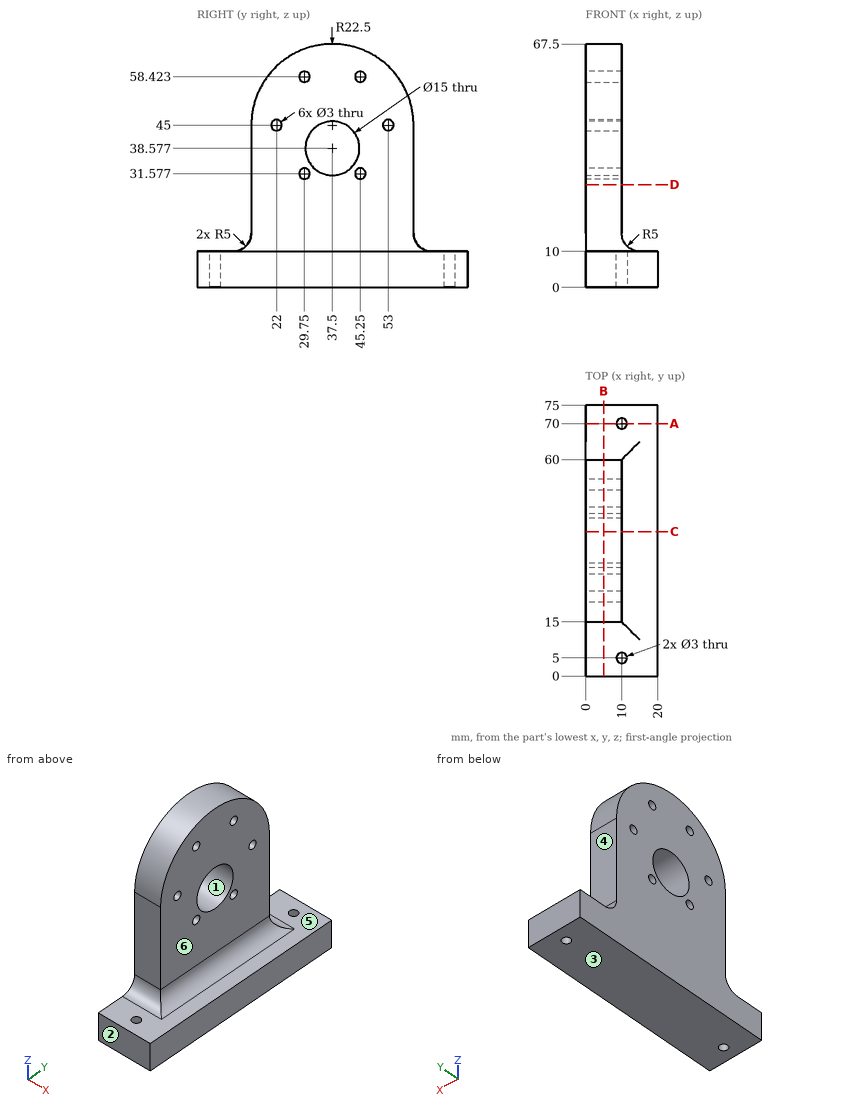
The drawing under review shows one solid part. Ordinate dimensions are in mm from its lowest x, y, z. A direction names the side the tool comes from. Round coordinates to 2 decimals unless told otherwise and drop trailing zeros. Loops run counter-clockwise (first coordinate to the right, second up) from the corner with the lowest first, then second, coordinate; pieces in that order, holes last. Notation, with made-up numbers: (13.5, 1) - (17.5, 1) arc R13 ccw to (17.5, 11) - close; hole circle Ø7 at (23, 87). An arc over 180 degrees is marked (long way). Put each result on its own line as item: value. Start each with the question number.
1. Insertion check: P1, Ø12, axis at y = 16.5, z = 32.5, coming from the +X side; P2, Ø1.5, axis at x = 5, y = 34.5, coming from the +Z side; P3, Ø6, axis at x = 9, z = 30, coming from the -Y side. Each pin has a flat end and moves straight along its axis. Give the tip position at first contact, or say it passes through.
2. Consider section A-A on y = 70. State the section outline as (x, z) points, plus the area to 3 significant figures.
3. Consider section C-C on y = 40. State the section outline as (x, z) points (1 decimal).
4. For the marked faces 4, 5 and 6, list the 3-axis set-ups (+Z, -Z, +X, -X, +Y, -Y) from which the entire face can be reached by the end or side of a thin tool; tool diameter is ignored.
5. Consider section B-B on x = 5. State the section outline as (y, z) points, plus the area to 3 significant figures.
6. Mouldability with a two-part tool opening along Z and no side actions: class the marked faces 1, 2 and 3 as +Z half, -Z half, draft (parallel to the pull), parting line (faces both ways), or undercut.
7. Consider section D-D on z = 28.5. State the section outline as (x, y) points, plus the area to 3 significant figures.
8. For probe 1 along Y at (x, z) = (10, 5.5); probe 2 along Y at (x, z) = (5.25, 45) (1 decimal); probe 3 along X at (y, z) = (70, 6.25), list the stretches that pass through material, from the lowest coordinate up. Write a range as [from, to].
Result sheet:
1. P1: x = 10
1. P2: z = 67.39
1. P3: y = 15
2. outline: (0, 0) - (8.5, 0) - (8.5, 10) - (0, 10) - close; (11.5, 0) - (20, 0) - (20, 10) - (11.5, 10) - close
2. area: 170 mm^2
3. outline: (0, 0) - (20, 0) - (20, 10) - (15, 10) arc R5 cw to (10, 15) - (10, 31.5) - (0, 31.5) - close; (0, 45.6) - (10, 45.6) - (10, 67.4) - (0, 67.4) - close
4. face 4: +Z, +X, -X, +Y
4. face 5: +Z, +X
4. face 6: +Z, +X, +Y, -Y
5. outline: (0, 0) - (75, 0) - (75, 10) - (65, 10) arc R5 cw to (60, 15) - (60, 45) arc R22.5 ccw to (15, 45) - (15, 15) arc R5 cw to (10, 10) - (0, 10) - close; hole circle Ø3 at (22, 45); hole circle Ø3 at (29.75, 31.58); hole circle Ø3 at (29.75, 58.42); hole circle Ø15 at (37.5, 38.58); hole circle Ø3 at (45.25, 31.58); hole circle Ø3 at (45.25, 58.42); hole circle Ø3 at (53, 45)
5. area: 2,910 mm^2
6. face 1: undercut
6. face 2: draft
6. face 3: -Z half
7. outline: (0, 15) - (10, 15) - (10, 60) - (0, 60) - close
7. area: 450 mm^2
8. probe 1: [0, 3.5], [6.5, 68.5], [71.5, 75]
8. probe 2: [15, 20.5], [23.5, 33.6], [41.4, 51.5], [54.5, 60]
8. probe 3: [0, 8.5], [11.5, 20]
